from build123d import *

# Parameters (mm, degrees)
SKETCH_R  = 4
PAD_DEPTH = 10


with BuildPart() as part:
    # Sketch → Pad (new body)
    with BuildSketch(Plane.YZ):
        Polygon((0, 0), (0, 66.568542), (-66.568542, 66.568542), (-66.568542, 56.568542), (-10, 0), align=None)
        with Locations((-14, 52.568542)):
            Circle(SKETCH_R, mode=Mode.SUBTRACT)
        with Locations((-52.568542, 52.568542)):
            Circle(SKETCH_R, mode=Mode.SUBTRACT)
        with Locations((-14, 14)):
            Circle(SKETCH_R, mode=Mode.SUBTRACT)
        with Locations((-33.285, 52.568542)):
            Circle(SKETCH_R, mode=Mode.SUBTRACT)
        with Locations((-14, 33.285)):
            Circle(SKETCH_R, mode=Mode.SUBTRACT)
        with Locations((-33.285, 33.285)):
            Circle(SKETCH_R, mode=Mode.SUBTRACT)
        with Locations((-42.9275, 42.9275)):
            Circle(SKETCH_R, mode=Mode.SUBTRACT)
        with Locations((-23.6425, 42.9275)):
            Circle(SKETCH_R, mode=Mode.SUBTRACT)
        with Locations((-23.6425, 23.6425)):
            Circle(SKETCH_R, mode=Mode.SUBTRACT)
    extrude(amount=PAD_DEPTH)


solid = part.part
The listing builds one solid part. Answer for the finished solid, in the listing's coordinates (mm). Coordinates: 2 decimals unless noted, no trailing zeros. Write each loop counter-clockwise with the first axis right and the second up, starting at its lowest first coordinate (ties: lowest second). Pieces come first, ordered by that corner, then holes. Notation, with made-up numbers: M 34,86 L 80,86 A16 cw 80,113 Z; hole C 52,11 d11. An arc over 180 degrees is marked long. Use one line per item in the form item = value.
Item 1: Find section B-B, the plane y = -14. Give the vertices of the cut face in (x, z) (3 decimals).
Model answer:
outline = M 0,4 L 10,4 L 10,10 L 0,10 Z; M 0,18 L 10,18 L 10,29.285 L 0,29.285 Z; M 0,37.285 L 10,37.285 L 10,48.569 L 0,48.569 Z; M 0,56.569 L 10,56.569 L 10,66.569 L 0,66.569 Z
Item 2: Find section A-A, the plane z = 14. Give the vertices of the cut face in (x, y).
Model answer:
outline = M 0,-24 L 10,-24 L 10,-18 L 0,-18 Z; M 0,-10 L 10,-10 L 10,0 L 0,0 Z
Item 3: Find section D-D, the plane x = 7. Give the number of separate pieces and of enclosed holes in the cut face, plus the area to 3 significant figures.
Model answer:
separate_pieces = 1
enclosed_holes = 9
area = 2,380 mm2
Item 4: The mould has two halves that part along Y. Classify faces 1 (the face through (5, -66.569, 62)), 2 (the face through (4.93, -24.51, 19.738)), 3 (the face through (10, -26, 49)): released by +Y, released by -Y, zero draft, split by the parting line, or undercut.
Model answer:
face_1 = released by -Y
face_2 = undercut
face_3 = zero draft
Item 5: Find section C-C, the plane y = -52. Give the vertices of the cut face in (x, z), plus the area to 3 significant figures.
Model answer:
outline = M 0,42 L 10,42 L 10,48.61 L 0,48.61 Z; M 0,56.53 L 10,56.53 L 10,66.57 L 0,66.57 Z
area = 166 mm2
Item 6: Find the intervals of material crossed by probe 1 along Z at (x, y) = (6.75, -14) (3 decimals); probe 2 along Y at (x, z) = (1, 35); probe 3 along Y at (x, z) = (9.75, 41), in increasing order.
Model answer:
probe_1 = 4 to 10, 18 to 29.285, 37.285 to 48.569, 56.569 to 66.569
probe_2 = -45 to -36.9, -29.67 to -17.61, -10.39 to 0
probe_3 = -51 to -46.43, -39.42 to -27.15, -20.14 to 0
Item 7: Given P1, Ø5, axis at x = 3, z = 40.5, coming from the -Y side, flat-ended and moving along its own axis, determine where the tip first touches the part or whether it passes through.
Model answer:
P1 = -53
